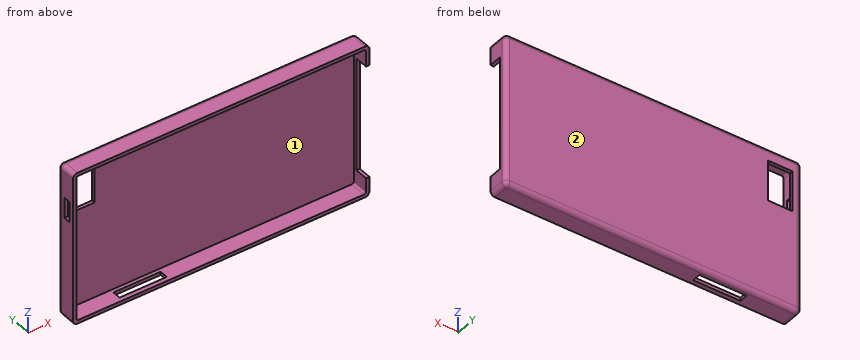
from build123d import *

# Parameters (mm, degrees)
F0_W      = 132
F0_H      = 68
F1_DEPTH  = 9
F2_T      = -1.5
F3_R      = 2
F4_W      = 3
F4_H      = 9
F5_DEPTH  = 25
F6_W      = 21
F6_H      = 3.811
F7_DEPTH  = 25
F8_W      = 11
F8_H      = 18
F9_DEPTH  = 25
F10_W     = 4.2909509502
F10_H     = 50.3760259598
F11_DEPTH = 25
F10_W_2   = 1.6166590303
F12_DEPTH = 5
F13_R     = 1


with BuildPart() as f1:
    # F0 (on Front) → F1 (new body)
    with BuildSketch(Plane.XZ):
        Rectangle(F0_W, F0_H)
    extrude(amount=F1_DEPTH)

    # F2
    f2_openings = [f1.faces().sort_by_distance(p)[0] for p in [
        (0, -9, 0),
    ]]
    offset(amount=F2_T, openings=f2_openings)

    # F3
    f3_edges = [f1.edges().sort_by_distance(p)[0] for p in [
        (-66, -4.5, -34),
        (0, 0, -34),
        (-66, 0, 0),
        (-66, -4.5, 34),
        (0, 0, 34),
        (66, 0, 0),
        (66, -4.5, -34),
        (66, -4.5, 34),
    ]]
    fillet(f3_edges, radius=F3_R)

    # F4 (on face) → F5 (cut)
    with BuildSketch(Plane(origin=(-66, 0, 0), x_dir=(0, -1, 0), z_dir=(-1, 0, 0))):
        with Locations((5.3369137328, 15.8999992609)):
            Rectangle(F4_W, F4_H)
    extrude(amount=-F5_DEPTH, mode=Mode.SUBTRACT)

    # F6 (on face) → F7 (cut)
    with BuildSketch(Plane(origin=(0, 0, -34), x_dir=(1, 0, 0), z_dir=(0, 0, -1))):
        with Locations((-33.2909998, 5.0821127795)):
            Rectangle(F6_W, F6_H)
    extrude(amount=-F7_DEPTH, mode=Mode.SUBTRACT)

    # F8 (on face) → F9 (cut)
    with BuildSketch(Plane.XZ):
        with Locations((-56.4135685265, 19.2365734056)):
            Rectangle(F8_W, F8_H)
    extrude(amount=F9_DEPTH, mode=Mode.SUBTRACT)

    # F10 (on face) → F11 (cut)
    with BuildSketch(Plane.YZ.offset(66)):
        with Locations((-5.2378654946, -0.4230095074)):
            Rectangle(F10_W, F10_H)
    extrude(amount=-F11_DEPTH, mode=Mode.SUBTRACT)

    # F10 (on face) → F12 (cut)
    with BuildSketch(Plane.YZ.offset(66)):
        with Locations((-8.1916704848, -0.4230095074)):
            Rectangle(F10_W_2, F10_H)
    extrude(amount=-F12_DEPTH, mode=Mode.SUBTRACT)

    # F13
    f13_edges = [f1.edges().sort_by_distance(p)[0] for p in [
        (-64.5, -5.25, 32.5),
        (-64.5, -5.25, -32.5),
        (64.5, -5.25, 32.5),
        (64.5, -5.25, -32.5),
    ]]
    fillet(f13_edges, radius=F13_R)


solid = f1.part
Geometry: final body of the model. Coordinates: model frame, mm. Face numbers are marked on the shaded views. Round coordinates to 2 decimals unless told otherwise and drop trailing zeros. Order: outer loops, then holes, each group sorted by start corner. A loop starts at its lowest first (then second) coordinate and runs counter-clockwise, first axis right, second up. Notation, with made-up numbers: (0.25, 12.5) -> (20.25, 12.5) arc R16 cw to (20.25, 31.5) -> close; hole circle Ø6 at (-39, -22). An arc over 180 degrees is marked (long way). Put each result on its own line as item: value. Start each with the question number.
Q1. Pull-direction query (Z, two-part tool) for the marked faces 1 and 2; classes: +Z half, -Z half, draft (parallel to the pull), parting line (faces both ways), or undercut.
Q2. Section B-B on x = -28. Return the cut outline in (y, z).
Q3. Section C-C on z = -9. Return the cut outline in (x, y), and give its area (3 significant figures).
Q4. Section A-A on z = 17.5. Return the cut outline in (x, y).
Q5. Line query: probe 1 along Z at (x, y) = (-7, -7.25); probe 2 along X at (y, z) = (-3.5, 30.5); probe 3 along X at (y, z) = (-4, -21). Output: solid intervals per line, ascending.
Q6. Section D-D on x = 53. Return the cut outline in (y, z).
Q7. First-contact query: pin 1 (0.8 mm diameter, centred on x = -65.5, z = 18, fed in from +Y); pin 2 (0.8 mm diameter, centred on x = -65.5, y = -5.5, fed in from -Z); pin 3 (4 mm diameter, centred on x = -39, z = -9, fed in from -Y). Flat tips, straight axial feed; report the tip coordinate or a pass-through.
Ans:
1. face 1: undercut
1. face 2: draft
2. outline: (-9, -34) -> (-6.99, -34) -> (-6.99, -32.5) -> (-9, -32.5) -> close; (-9, 32.5) -> (-1.5, 32.5) -> (-1.5, -32.5) -> (-3.18, -32.5) -> (-3.18, -34) -> (-2, -34) arc R2 ccw to (0, -32) -> (0, 32) arc R2 ccw to (-2, 34) -> (-9, 34) -> close
3. outline: (-66, -9) -> (-64.5, -9) -> (-64.5, -1.5) -> (64.5, -1.5) -> (64.5, -3.09) -> (66, -3.09) -> (66, -2) arc R2 ccw to (64, 0) -> (-64, 0) arc R2 ccw to (-66, -2) -> close
3. area: 210 mm2
4. outline: (-66, -9) -> (-64.5, -9) -> (-64.5, -6.84) -> (-66, -6.84) -> close; (-66, -3.84) -> (-64.5, -3.84) -> (-64.5, -1.5) -> (-61.91, -1.5) -> (-61.91, 0) -> (-64, 0) arc R2 ccw to (-66, -2) -> close; (-50.91, -1.5) -> (64.5, -1.5) -> (64.5, -3.09) -> (66, -3.09) -> (66, -2) arc R2 ccw to (64, 0) -> (-50.91, 0) -> close
5. probe 1: z = -34 to -32.5, 32.5 to 34
5. probe 2: x = -66 to -64.5, 64.5 to 66
5. probe 3: x = -66 to -64.5
6. outline: (-9, -34) -> (-2, -34) arc R2 ccw to (0, -32) -> (0, 32) arc R2 ccw to (-2, 34) -> (-9, 34) -> (-9, 32.5) -> (-1.5, 32.5) -> (-1.5, -32.5) -> (-9, -32.5) -> close
7. pin 1: stops at y = -0.33
7. pin 2: stops at z = -33.67
7. pin 3: stops at y = -1.5
